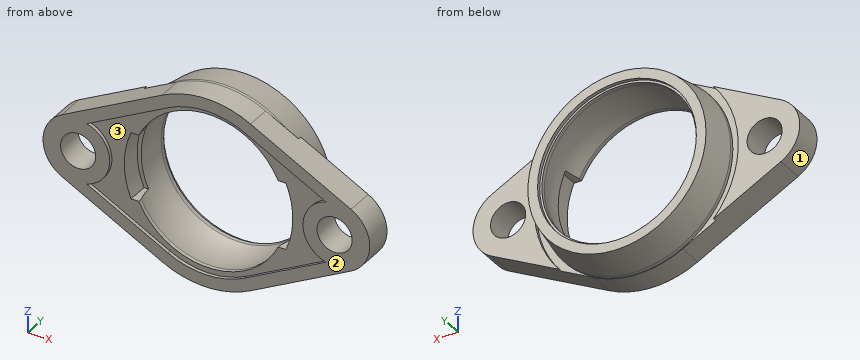
```python
from build123d import *

# Parameters (mm, degrees)
SKETCH1_R              = 11
FLANGE_DEPTH           = 4
SKETCH3_R              = 13.425
TOP_RECESS_DEPTH       = 0.5
BOTTOM_RECESS_1_DEPTH  = 0.5
BOTTOM_RECESS_2_DEPTH  = 3
MOUNTING_HOLE_M5X0_8_D = 5


with BuildPart() as part:
    # Sketch1 → Flange (new body)
    with BuildSketch(Plane(origin=(0, 0, 0), x_dir=(1, 0, 0), z_dir=(0, 1, 0))):
        with BuildLine():
            Line((20.578767123, 4.424572712), (6.287671233, 11.946346323))
            ThreePointArc((6.287671233, 11.946346323), (0, 13.5), (-6.287671233, 11.946346323))
            Line((-6.287671233, 11.946346323), (-20.578767123, 4.424572712))
            ThreePointArc((-20.578767123, 4.424572712), (-23.25, 0), (-20.578767123, -4.424572712))
            Line((-20.578767123, -4.424572712), (-6.287671233, -11.946346323))
            ThreePointArc((-6.287671233, -11.946346323), (0, -13.5), (6.287671233, -11.946346323))
            Line((6.287671233, -11.946346323), (20.578767123, -4.424572712))
            ThreePointArc((20.578767123, -4.424572712), (23.25, 0), (20.578767123, 4.424572712))
        make_face()
        Circle(SKETCH1_R, mode=Mode.SUBTRACT)
    extrude(amount=FLANGE_DEPTH)

    # Sketch2 → Bearing Seat (revolve)
    with BuildSketch(Plane.XY):
        Polygon((-13.425, 4), (-12.675, 8.5), (-11.3, 8.5), (-11.3, 8), (-11, 8), (-11, 4), align=None)
    revolve(axis=Axis((0, 0, 0), (0, 1, 0)))

    # Sketch3 → Top Recess (cut)
    with BuildSketch(Plane(origin=(0, 4, 0), x_dir=(1, 0, 0), z_dir=(0, 1, 0))):
        with BuildLine():
            Line((10.970198855, 9.481810855), (6.287671233, 11.946346323))
            ThreePointArc((6.287671233, 11.946346323), (0, 13.5), (-6.287671233, 11.946346323))
            Line((-6.287671233, 11.946346323), (-10.970198855, 9.481810855))
            ThreePointArc((-10.970198855, 9.481810855), (-14.5, 0), (-10.970198855, -9.481810855))
            Line((-10.970198855, -9.481810855), (-6.287671233, -11.946346323))
            ThreePointArc((-6.287671233, -11.946346323), (0, -13.5), (6.287671233, -11.946346323))
            Line((6.287671233, -11.946346323), (10.970198855, -9.481810855))
            ThreePointArc((10.970198855, -9.481810855), (14.5, 0), (10.970198855, 9.481810855))
        make_face()
        Circle(SKETCH3_R, mode=Mode.SUBTRACT)
    extrude(amount=-TOP_RECESS_DEPTH, mode=Mode.SUBTRACT)

    # Sketch5 → Bottom Recess 1 (cut)
    with BuildSketch(Plane.XZ):
        with BuildLine():
            Line((17.009424329, 4.325618107), (5.47260274, 10.397745874))
            ThreePointArc((5.47260274, 10.397745874), (0, 11.75), (-5.47260274, 10.397745874))
            Line((-5.47260274, 10.397745874), (-17.009424329, 4.325618107))
            ThreePointArc((-17.009424329, 4.325618107), (-13.75, 0), (-17.009424329, -4.325618107))
            Line((-17.009424329, -4.325618107), (-5.47260274, -10.397745874))
            ThreePointArc((-5.47260274, -10.397745874), (0, -11.75), (5.47260274, -10.397745874))
            Line((5.47260274, -10.397745874), (17.009424329, -4.325618107))
            ThreePointArc((17.009424329, -4.325618107), (13.75, 0), (17.009424329, 4.325618107))
        make_face()
    extrude(amount=-BOTTOM_RECESS_1_DEPTH, mode=Mode.SUBTRACT)

    # Sketch6 → Bottom Recess 2 (cut)
    with BuildSketch(Plane.XZ.offset(-0.5)):
        with BuildLine():
            Line((-11.01986842, 4.75), (11.01986842, 4.75))
            ThreePointArc((11.01986842, 4.75), (12, 0), (11.01986842, -4.75))
            Line((11.01986842, -4.75), (-11.01986842, -4.75))
            ThreePointArc((-11.01986842, -4.75), (-12, 0), (-11.01986842, 4.75))
        make_face()
    extrude(amount=-BOTTOM_RECESS_2_DEPTH, mode=Mode.SUBTRACT)

    # Mounting Hole _M5x0.8 (through all)
    with Locations(Plane(origin=(0, 4, 0), x_dir=(1, 0, 0), z_dir=(0, 1, 0))):
        with Locations((18.25, 0), (-18.25, 0)):
            Hole(MOUNTING_HOLE_M5X0_8_D / 2)

    # Sketch11 → Cut-Revolve1 (revolve, cut)
    with BuildSketch(Plane.XY):
        with BuildLine():
            Line((0, 15.70600279), (0, -7.20600279))
            ThreePointArc((0, -7.20600279), (11.45600279, 4.25), (0, 15.70600279))
        make_face()
    revolve(axis=Axis((0, 8.5, 0), (0, -1, 0)), mode=Mode.SUBTRACT)


solid = part.part
```
Verification items for the finished model (mm, model axes). Face numbers are marked on the shaded views. Give positions to 0.01 mm unless a question says otherwise; leave off trailing zeros. Order: outer loops, then holes, each group sorted by start corner. A loop starts at its lowest first (then second) coordinate and runs counter-clockwise, first axis right, second up. Notation, with made-up numbers: (-35.75, 48) -> (20.25, 48) arc R16 cw to (20.25, 79) -> close; hole circle Ø4 at (-35, -5). An arc over 180 degrees is marked (long way). One line per item, written item: value.
(1) Sectioned sample at A-A on x = 0. Record the cut outline in (y, z) (3 decimals), then the cut area to 3 significant figures.
Final values:
outline: (0, -13.5) -> (3.5, -13.5) -> (3.5, -13.425) -> (4, -13.425) -> (8.5, -12.675) -> (8.5, -11.3) -> (8, -11.3) -> (8, -11) -> (7.45, -11) arc R11.456 cw to (1.05, -11) -> (0.5, -11) -> (0.5, -11.75) -> (0, -11.75) -> close; (0, 11.75) -> (0.5, 11.75) -> (0.5, 11) -> (1.05, 11) arc R11.456 cw to (7.45, 11) -> (8, 11) -> (8, 11.3) -> (8.5, 11.3) -> (8.5, 12.675) -> (4, 13.425) -> (3.5, 13.425) -> (3.5, 13.5) -> (0, 13.5) -> close
area: 33.4 mm^2
(2) Scan lines: line 1 along X through (y, z) = (2.25, -2); line 2 along Z through (x, y) = (4, 5.5); line 3 along Z through (x, y) = (-2.5, 7). Record each from-to range of solid material in increasing order. Write a range as [from, to].
Final values:
line 1: [-22.83, -19.75], [-16.75, -11.83], [11.83, 16.75], [19.75, 22.83]
line 2: [-12.55, -10.66], [10.66, 12.55]
line 3: [-12.68, -10.84], [10.84, 12.68]
(3) Sectioned sample at C-C on z = 0. Count the separate pieces of the cut face and the enclosed holes in it, then the cut area to 3 significant figures.
Final values:
separate pieces: 4
enclosed holes: 0
area: 63.7 mm^2
(4) Draft check along Z on the marked faces 1, 2 and 3. Enter one of: pulls with the +Z half, pulls with the -Z half, needs draft (parallel to the pull), parting line crosses it, or undercut.
Final values:
face 1: parting line crosses it
face 2: needs draft
face 3: undercut
(5) Sectioned sample at B-B on y = 2. Record the cut outline in (x, z), then the cut area to 3 significant figures.
Final values:
outline: (-20.58, -4.42) -> (-6.29, -11.95) arc R13.5 ccw to (6.29, -11.95) -> (20.58, -4.42) arc R5 ccw to (20.58, 4.42) -> (6.29, 11.95) arc R13.5 ccw to (-6.29, 11.95) -> (-20.58, 4.42) arc R5 ccw to start; hole circle Ø5 at (-18.25, 0); hole (-11.02, -4.75) -> (-10.18, -4.75) arc R11.23 ccw to (10.18, -4.75) -> (11.02, -4.75) arc R12 ccw to (11.02, 4.75) -> (10.18, 4.75) arc R11.23 ccw to (-10.18, 4.75) -> (-11.02, 4.75) arc R12 ccw to start; hole circle Ø5 at (18.25, 0)
area: 378 mm^2
(6) Gauge pin test, flat ends, axial feed: pin 1 (6 mm diameter, centred on x = 18.25, z = 0, fed in from +Y); pin 2 (2 mm diameter, centred on x = 15.5, z = 8.5, fed in from +Y); pin 3 (1.8 mm diameter, centred on x = -11.5, z = -2, fed in from -Y); pin 4 (1.2 mm diameter, centred on x = 10.5, y = 2.5, fed in from -Z). Record the tip position at first contact, or that the pin passes through.
Final values:
pin 1: y = 4
pin 2: through
pin 3: y = 0.5
pin 4: z = -10.05
(7) Sectioned sample at D-D on x = -18.25. Record the cut outline in (y, z).
Final values:
outline: (0, -5.65) -> (4, -5.65) -> (4, -2.5) -> (0, -2.5) -> close; (0, 2.5) -> (4, 2.5) -> (4, 5.65) -> (0, 5.65) -> close
